Part print with two shaded views. Sizes in mm from the minimum x, y, z corner. A direction names the side the tool comes from. Round coordinates to 2 decimals unless told otherwise and drop trailing zeros. Write each loop counter-clockwise with the first axis right and the second up, starting at its lowest first coordinate (ties: lowest second). Pieces come first, ordered by that corner, then holes. Notation, with made-up numbers: (15, 73) - (45, 73) arc R15 cw to (45, 95) - close; hole circle Ø8 at (68.5, 48.5). An arc over 180 degrees is marked (long way). Answer as a JSON object with one key per item and string values. Group by question number.
Item 1: Two-plate mould, pull along Y, no slides. Class the marked faces 1, 2 and 3: +Y half, -Y half, draft (parallel to the pull), parting line (faces both ways), or undercut.
Item 2: Slice it at A-A, the plane z = 73.5. List the corners of the cut face in (x, y), then the cut area to 3 significant figures.
Item 3: Slice it at B-B, the plane y = 55. List the corners of the cut face in (x, z).
Item 4: Probe line 1 (X direction, y = 115.5, z = 6.5); line 2 (Y direction, x = 65, z = 68). List the from-to ranges inside material, lowest first. Write a range as from..to.
Item 5: Flat gauge pins, fed straight in: pin 1 (8 mm diameter, centred on x = 54, z = 60, fed in from -Y); pin 2 (2.5 mm diameter, centred on x = 65, y = 65, fed in from +Z). Where does each tip first touch, or does it go through?
Item 6: Which spindle directions (+Z, -Z, +X, -X, +Y, -Y) get a long thin tool onto all of the face, cutting with end or side? Do the marked faces 4 and 5. Say none if no direction does.
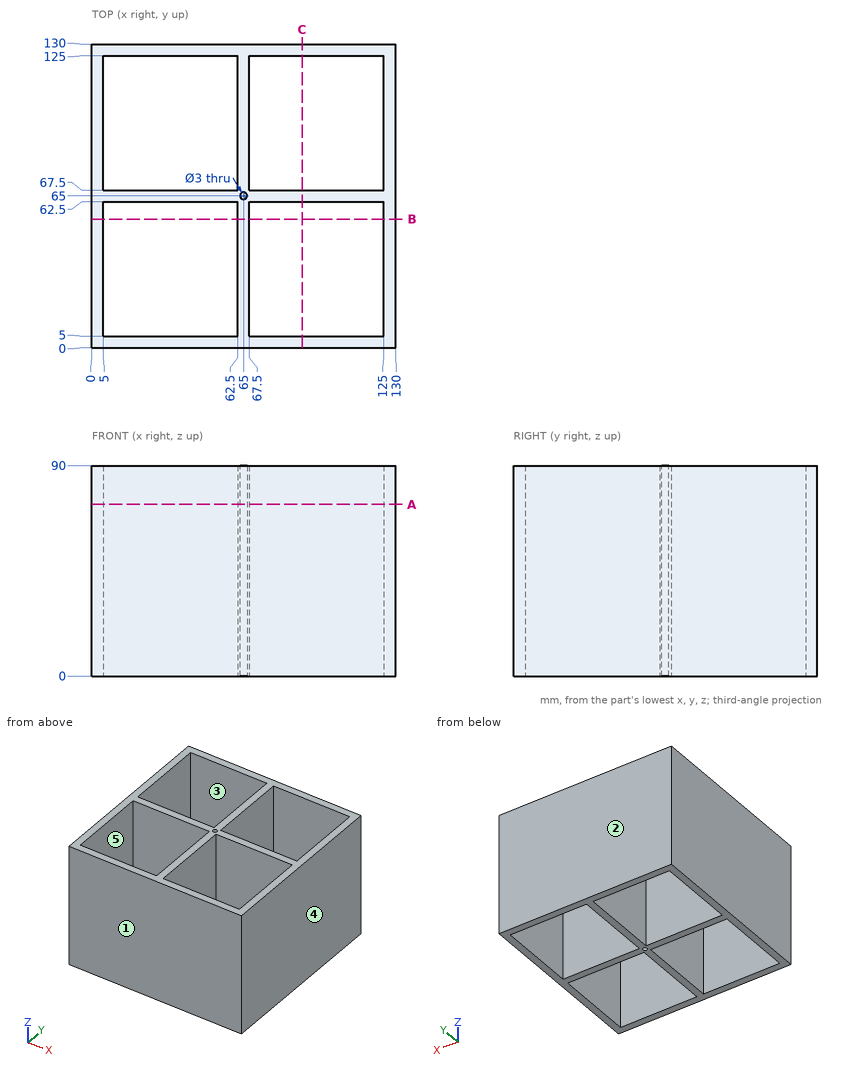
Geometry says:
{
 "1": {"face 1": "-Y half", "face 2": "+Y half", "face 3": "undercut"},
 "2": {"outline": "(0, 0) - (130, 0) - (130, 130) - (0, 130) - close; hole (5, 5) - (62.5, 5) - (62.5, 62.5) - (5, 62.5) - close; hole (5, 67.5) - (62.5, 67.5) - (62.5, 125) - (5, 125) - close; hole circle Ø3 at (65, 65); hole (67.5, 5) - (125, 5) - (125, 62.5) - (67.5, 62.5) - close; hole (67.5, 67.5) - (125, 67.5) - (125, 125) - (67.5, 125) - close", "area": "3,670 mm^2"},
 "3": {"outline": "(0, 0) - (5, 0) - (5, 90) - (0, 90) - close; (62.5, 0) - (67.5, 0) - (67.5, 90) - (62.5, 90) - close; (125, 0) - (130, 0) - (130, 90) - (125, 90) - close"},
 "4": {"line 1": "x = 0..5, 62.5..67.5, 125..130", "line 2": "y = 0..63.5, 66.5..130"},
 "5": {"pin 1": "stops at y = 0", "pin 2": "passes through"},
 "6": {"face 4": "+Z, -Z, +X, +Y, -Y", "face 5": "+Z, -Z"}
}
